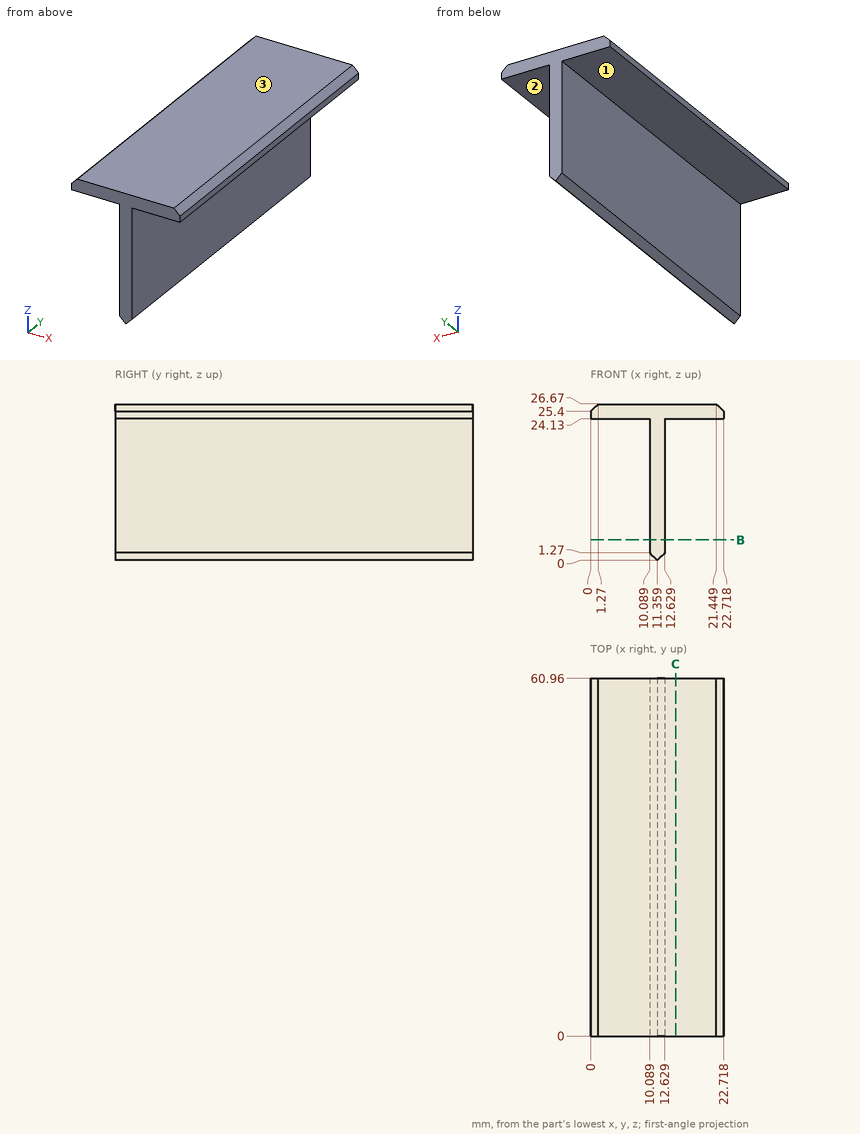
Could you check a few things on this drawing? It's one solid part, dimensions in mm from its lowest x, y, z. A direction names the side the tool comes from. Coordinates: 2 decimals unless noted, no trailing zeros. Order: outer loops, then holes, each group sorted by start corner. A loop starts at its lowest first (then second) coordinate and runs counter-clockwise, first axis right, second up.
1) Which directions (+Z, -Z, +X, -X, +Y, -Y) give clear straight access to the entire face, cutting with the end or side of a thin tool? Please do the marked faces 1, 2 and 3.
2) I need wall thicknesses on line 1 (X direction, y = 17, z = 21); line 2 (Z direction, x = 2, y = 3.5); line 3 (Z direction, x = 1, y = 52). Which ranges of each line are inside material? Lowest first, please.
3) Imagine slicing it at C-C on x = 14.5. List the corners of the cut face in (y, z) for me.
4) Will these pins go through, and if not, where does the flat tip stop? pin 1 (5 mm diameter, centred on x = 5.5, y = 26.5, fed in from -Z); pin 2 (4 mm diameter, centred on y = 24.5, z = 18.5, fed in from +X); pin 3 (10 mm diameter, centred on y = 53, z = 11, fed in from -X).
5) Imagine slicing it at B-B on z = 3.5. List the corners of the cut face in (x, y) for me, and give its area (3 significant figures).
Response values:
1. face 1: -Z, -X, +Y, -Y
1. face 2: -Z, +X, +Y, -Y
1. face 3: +Z, +X, -X, +Y, -Y
2. line 1: x = 10.09 to 12.63
2. line 2: z = 24.13 to 26.67
2. line 3: z = 24.13 to 26.4
3. outline: (0, 24.13) - (60.96, 24.13) - (60.96, 26.67) - (0, 26.67) - close
4. pin 1: stops at z = 24.13
4. pin 2: stops at x = 12.63
4. pin 3: stops at x = 10.09
5. outline: (10.09, 0) - (12.63, 0) - (12.63, 60.96) - (10.09, 60.96) - close
5. area: 155 mm2
